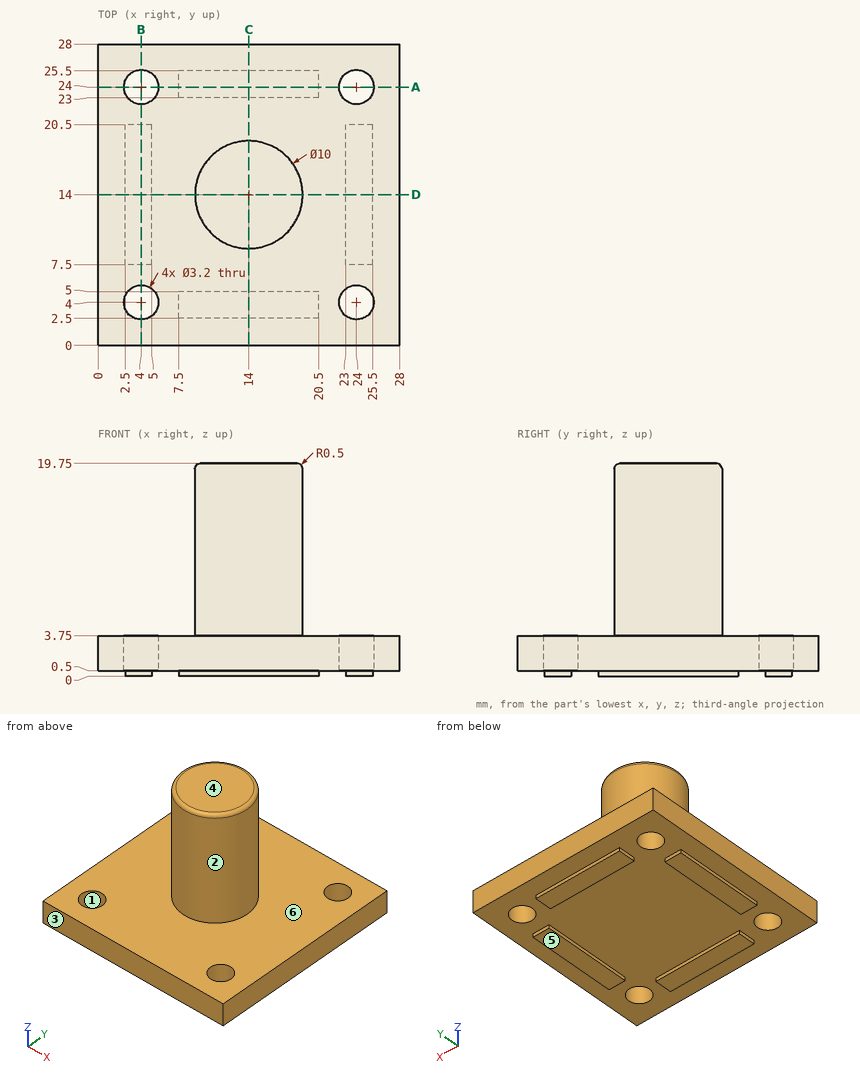
For this review, use the dimensioned drawing (mm, ordinates from the lowest corner) and the shaded views. A direction names the side the tool comes from. Give positions to 0.01 mm unless a question says otherwise; leave off trailing zeros. Write each loop counter-clockwise with the first axis right and the second up, starting at its lowest first coordinate (ties: lowest second). Pieces come first, ordered by that corner, then holes. Notation, with made-up numbers: M 4.5,-19.5 L 17.5,-19.5 A12 ccw 17.5,-14.5 Z; hole C 18,61 d9. An arc over 180 degrees is marked long. Answer as a JSON object with one key per item and string values. Group by question number.
Item 1: For probe 1 along Y at (x, z) = (24, 3.1); probe 2 along Z at (x, y) = (23.5, 22); probe 3 along Z at (x, y) = (14.25, 16.25), list the stretches that pass through material, from the lowest coordinate up. Write a range as [from, to].
Item 2: Tool access review of the marked faces 5 and 6: name each direction out of +Z, -Z, +X, -X, +Y, -Y from which nothing blocks a thin tool from reaching the whole face with its end or side.
Item 3: Draft analysis for pull direction Y (two halves, no side actions). For the marked faces 1, 2, 3 and 4, state which applies: +Y half, -Y half, draft (parallel to the pull), parting line (faces both ways), or undercut.
Item 4: Consider section A-A on y = 24. Write out the cut boundary in (x, z).
Item 5: Consider section C-C on x = 14. Write out the cut boundary in (y, z), plus the area to 3 significant figures.
Item 6: For pin 1 Ø4 at (y, z) = (19.5, 12.5) entering from -X; pin 2 Ø5 at (x, y) = (4, 4) entering from -Z; pin 3 Ø1 at (x, z) = (13, 7) entering from -Y; pin 4 Ø10 at (y, z) = (3, 5.5) entering from -X, all flat-tipped, find the tip position at first contact; note any pin that passes through.
Check result:
{
 "1": {"probe 1": "y = [0, 2.4], [5.6, 22.4], [25.6, 28]", "probe 2": "z = [0.5, 3.75]", "probe 3": "z = [0.5, 19.75]"},
 "2": {"face 5": "-Z, +X, -X, +Y, -Y", "face 6": "+Z"},
 "3": {"face 1": "undercut", "face 2": "parting line", "face 3": "-Y half", "face 4": "draft"},
 "4": {"outline": "M 0,0.5 L 2.4,0.5 L 2.4,3.75 L 0,3.75 Z; M 5.6,0.5 L 7.5,0.5 L 7.5,0 L 20.5,0 L 20.5,0.5 L 22.4,0.5 L 22.4,3.75 L 5.6,3.75 Z; M 25.6,0.5 L 28,0.5 L 28,3.75 L 25.6,3.75 Z"},
 "5": {"outline": "M 0,0.5 L 2.5,0.5 L 2.5,0 L 5,0 L 5,0.5 L 23,0.5 L 23,0 L 25.5,0 L 25.5,0.5 L 28,0.5 L 28,3.75 L 19,3.75 L 19,19.25 A0.5 ccw 18.5,19.75 L 9.5,19.75 A0.5 ccw 9,19.25 L 9,3.75 L 0,3.75 Z", "area": "253 mm^2"},
 "6": {"pin 1": "stops at x = 10.43", "pin 2": "stops at z = 0.5", "pin 3": "stops at y = 9.03", "pin 4": "stops at x = 0"}
}
